Drawing for the job (mm, zero at the part's lowest x, y, z). Give positions to 0.01 mm unless a question says otherwise; leave off trailing zeros. Loops run counter-clockwise (first coordinate to the right, second up) from the corner with the lowest first, then second, coordinate; pieces in that order, holes last. Notation, with made-up numbers: (-32.75, -33) - (12.25, -33) arc R12 cw to (12.25, -22) - close; hole circle Ø11 at (68.5, 69). An arc over 180 degrees is marked (long way). Return JSON: item names as keys, results as strings. Group by question number.
1) Slice it at B-B (x = 12.5). List the corners of the cut face in (y, z).
2) Drill centre lines: probe 1 along Y at (x, z) = (12.5, 0.75); probe 2 along X at (y, z) = (9, 0.4). Where is each one in solid material? Low to high. Write a range as from..to.
3) Slice it at C-C (y = 10). List the corners of the cut face in (x, z).
4) Slice it at A-A (z = 1.6). List the corners of the cut face in (x, y), and give its area (3 significant figures).
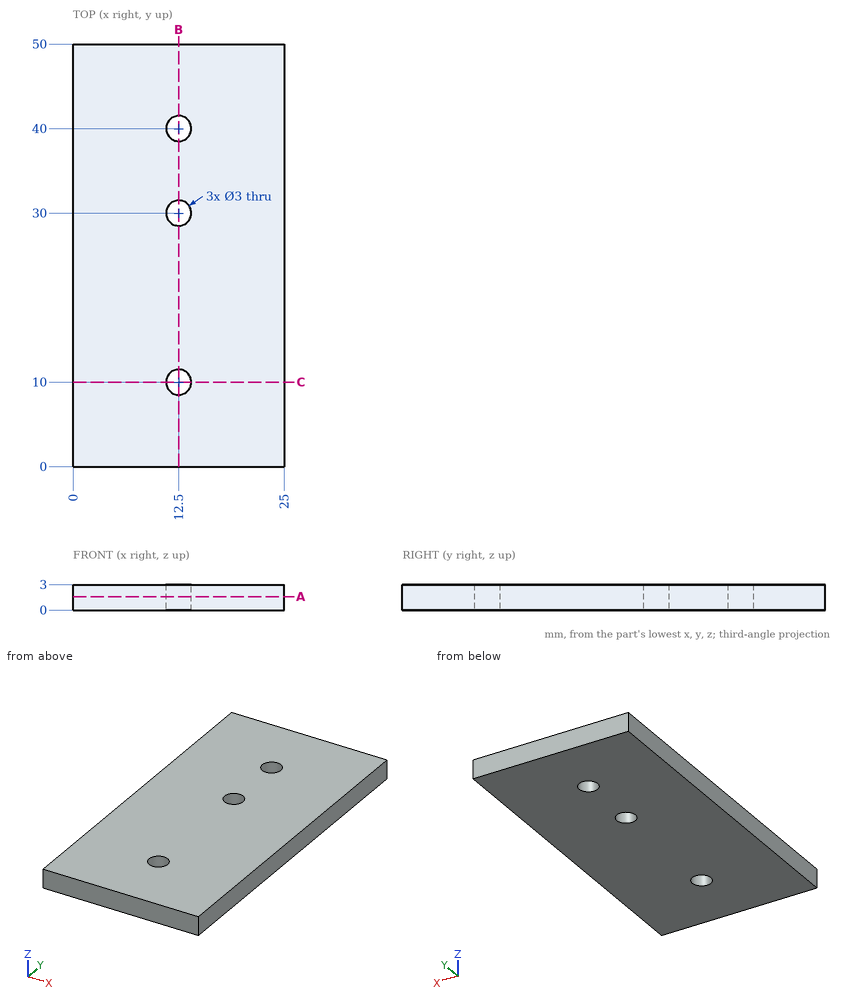
Results:
{
 "1": {"outline": "(0, 0) - (8.5, 0) - (8.5, 3) - (0, 3) - close; (11.5, 0) - (28.5, 0) - (28.5, 3) - (11.5, 3) - close; (31.5, 0) - (38.5, 0) - (38.5, 3) - (31.5, 3) - close; (41.5, 0) - (50, 0) - (50, 3) - (41.5, 3) - close"},
 "2": {"probe 1": "0..8.5, 11.5..28.5, 31.5..38.5, 41.5..50", "probe 2": "0..11.38, 13.62..25"},
 "3": {"outline": "(0, 0) - (11, 0) - (11, 3) - (0, 3) - close; (14, 0) - (25, 0) - (25, 3) - (14, 3) - close"},
 "4": {"outline": "(0, 0) - (25, 0) - (25, 50) - (0, 50) - close; hole circle Ø3 at (12.5, 10); hole circle Ø3 at (12.5, 30); hole circle Ø3 at (12.5, 40)", "area": "1,230 mm2"}
}
